Source: CAD feature listing. Evaluate the final solid. Frame: model axes, mm. Face numbers are marked on the shaded views. A direction names the side the tool comes from. Coordinates: 2 decimals unless noted, no trailing zeros. Order: outer loops, then holes, each group sorted by start corner. A loop starts at its lowest first (then second) coordinate and runs counter-clockwise, first axis right, second up. Notation, with made-up numbers: (-19, -8) - (-2, -8) arc R15 ccw to (-2, 4) - close; hole circle Ø2 at (3, -4.5). An arc over 180 degrees is marked (long way). One line per question, with ' | ' between items.
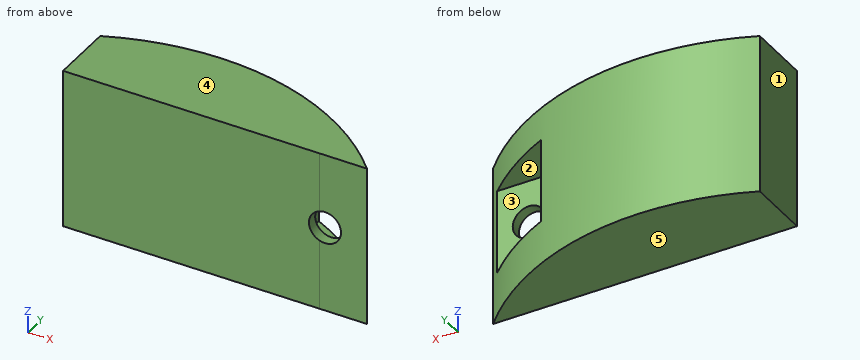
Autodesk Inventor part; units mm, degrees
ref_plane "РабПлоскость1" through (10.0583, 2.1127, 0) normal (0, -1, 0) x (1, 0, 0)
ref_plane "YZ Plane" through (0, 0, 0) normal (1, 0, 0) x (0, 1, 0)
ref_plane "XZ Plane" through (0, 0, 0) normal (0, 1, 0) x (-1, 0, 0)
sketch "Эскиз1" plane through (0, 0, 0) normal (0, 0, 1) x (1, 0, 0)
  arc A0 (28.4298, -5.9319) -> (0, 0) centre (10.0583, -22.8873) ccw
  line L0 (0, -5.9315) -> (0, 0)
  line L1 (23.9975, -5.9315) -> (0, -5.9315)
  line L2 (23.9975, -5.9315) -> (23.998, -5.9315)
  line L3 (23.998, -5.9319) -> (23.998, -5.9315)
  line L4 (23.998, -5.9319) -> (28.4298, -5.9319)
  point P0 (0, 0)
  point P1 (-10.0583, 22.8873)
extrude "Выдавливание1" add sketch "Эскиз1" along normal blind 15
ref_plane "РабПлоскость1" through (10.0583, 2.1127, 0) normal (0, -1, 0) x (1, 0, 0)
sketch "Эскиз2" plane through (10.0583, 2.1127, 0) normal (0, -1, 0) x (1, 0, 0)
  circle A0 centre (14.4417, 8) radius 1.5
  line L0 (18.3715, 0) -> (18.3715, 15)
  line L1 (10.5118, 11.93) -> (18.3715, 11.93)
  line L2 (18.3715, 11.93) -> (18.3715, 4.07)
  line L3 (18.3715, 4.07) -> (10.5118, 4.07)
  line L4 (10.5118, 4.07) -> (10.5118, 11.93)
  line L5 (10.5118, 11.93) -> (18.3715, 4.07) construction
  line L6 (18.3715, 11.93) -> (10.5118, 4.07) construction
  point P0 (-10.0583, 0)
  dimension "d2" = 7.86
extrude "Выдавливание2" cut sketch "Эскиз2" along normal blind 10.2942 contours A0
sketch "Эскиз3" plane through (10.0583, 2.1127, 0) normal (0, -1, 0) x (1, 0, 0)
  circle A0 centre (14.4417, 8) radius 1.5
  line L0 (18.3715, 0) -> (18.3715, 15)
  line L1 (10.5118, 11.93) -> (18.3715, 11.93)
  line L2 (18.3715, 11.93) -> (18.3715, 4.07)
  line L3 (18.3715, 4.07) -> (10.5118, 4.07)
  line L4 (10.5118, 4.07) -> (10.5118, 11.93)
  line L5 (10.5118, 11.93) -> (18.3715, 4.07) construction
  line L6 (18.3715, 11.93) -> (10.5118, 4.07) construction
  point P0 (-10.0583, 0)
  point P1 (-10.0583, 0)
  dimension "d5" = 7.86
extrude "Выдавливание3" cut sketch "Эскиз3" along normal blind 7.0442
properties part number "KB33-046-002-006 - Заглушка"
(1) Cut plane D-D (x = 24.5). Return the cut outline in (y, z).
Taken from the geometry:
outline: (-5.93, 0) - (-2.48, 0) - (-2.48, 4.07) - (-4.93, 4.07) - (-4.93, 6.5) - (-5.93, 6.5) - close; (-5.93, 9.5) - (-4.93, 9.5) - (-4.93, 11.93) - (-2.48, 11.93) - (-2.48, 15) - (-5.93, 15) - close
(2) Material intervals for L1, parallel to Z at x = 24.5, y = -5.15; L2, parallel to X at y = -0.5, z = 11; L3, parallel to Y at x = 20.75, z = 7.75, sorted ascending. Write a range as from..to.
Taken from the geometry:
L1: z = 0..6.5, 9.5..15 | L2: x = 0..20.57 | L3: y = -5.93..-4.93
(3) Cut plane B-B (y = -1.75). Return the cut outline in (x, z), and give its area (3 significant figures).
Taken from the geometry:
outline: (0, 0) - (23.41, 0) - (23.41, 4.07) - (20.57, 4.07) - (20.57, 11.93) - (23.41, 11.93) - (23.41, 15) - (0, 15) - close | area: 329 mm²
(4) Cut plane A-A (z = 8). Return the cut outline in (x, y).
Taken from the geometry:
outline: (0, -5.93) - (23, -5.93) - (23, -4.93) - (20.57, -4.93) - (20.57, -0.2) arc R25 ccw to (0, 0) - close; (26, -5.93) - (28.43, -5.93) arc R25 ccw to (27.45, -4.93) - (26, -4.93) - close
(5) Set-up query: the marked faces 1 and 2. Return all of +Z, -Z, +X, -X, +Y, -Y with unobstructed straight access to the full face (end or side cutting, diameter ignored); none if empty.
Taken from the geometry:
face 1: +Z, -Z, -X, +Y, -Y | face 2: +X, +Y
(6) Cut plane C-C (z = 11.25). Return the cut outline in (x, y), and give its area (3 significant figures).
Taken from the geometry:
outline: (0, -5.93) - (24, -5.93) - (28.43, -5.93) arc R25 ccw to (27.45, -4.93) - (20.57, -4.93) - (20.57, -0.2) arc R25 ccw to (0, 0) - close | area: 158 mm²
(7) Pull-direction query (Z, two-part tool) for the marked faces 3, 4 and 5; classes: pulls with the +Z half, pulls with the -Z half, needs draft (parallel to the pull), parting line crosses it, or undercut.
Taken from the geometry:
face 3: undercut | face 4: pulls with the +Z half | face 5: pulls with the -Z half
(8) Pin query (flat end, axial travel): P1, Ø1, axis at x = 10, y = -1, coming from the -Z side; P2, Ø3.5, axis at x = 24.5, z = 9, coming from the +Y side; P3, Ø1, axis at y = 0.5, z = 8, coming from the +X side. Return the tip coordinate at first contact, or that it passes through.
Taken from the geometry:
P1: stops at z = 0 | P2: stops at y = -4.93 | P3: stops at x = 20.12
